Here's how the part is built. I have some questions about the finished solid (model axes, mm). Coordinates: 2 decimals unless noted, no trailing zeros. Order: outer loops, then holes, each group sorted by start corner. A loop starts at its lowest first (then second) coordinate and runs counter-clockwise, first axis right, second up. Notation, with made-up numbers: (17, 9) - (57, 9) arc R18 cw to (57, 27) - close; hole circle Ø1 at (46.25, 73.25). An arc over 180 degrees is marked (long way). Use one line per item in the form item = value. Start each with the question number.
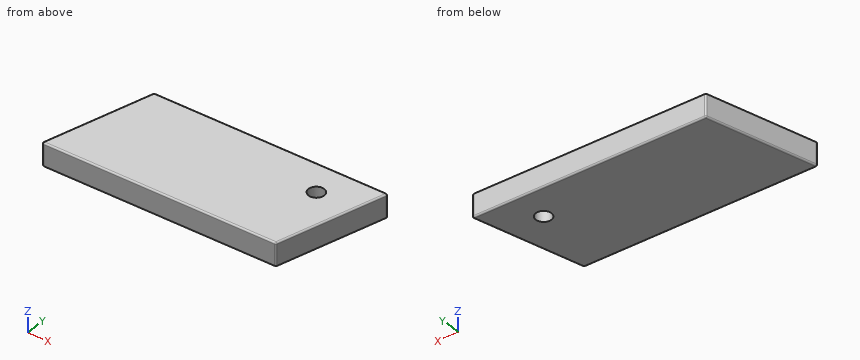
from build123d import *

# Parameters (mm, degrees)
BOSS_EXTRUDE1_DEPTH = 19.05
SKETCH2_R           = 6.35
CUT_EXTRUDE1_DEPTH  = 19.05
FILLET1_R           = 1.27


with BuildPart() as part:
    # Sketch1 → Boss-Extrude1 (new body)
    with BuildSketch(Plane.XY):
        Polygon((0, 0), (23.820683207, 88.9), (214.320683207, 88.9), (190.5, 0), align=None)
    extrude(amount=BOSS_EXTRUDE1_DEPTH)

    # Sketch2 → Cut-Extrude1 (cut)
    with BuildSketch(Plane.XY.offset(19.05)):
        with Locations((176.220683207, 62.083789013)):
            Circle(SKETCH2_R)
    extrude(amount=-CUT_EXTRUDE1_DEPTH, mode=Mode.SUBTRACT)

    # Fillet1
    fillet1_edges = [part.edges().sort_by_distance(p)[0] for p in [
        (119.070683207, 88.9, 19.05),
        (11.910341604, 44.45, 19.05),
        (95.25, 0, 19.05),
        (11.910341604, 44.45, 0),
        (119.070683207, 88.9, 0),
        (202.410341604, 44.45, 0),
        (95.25, 0, 0),
        (0, 0, 9.525),
        (23.820683207, 88.9, 9.525),
        (214.320683207, 88.9, 9.525),
        (190.5, 0, 9.525),
        (202.410341604, 44.45, 19.05),
    ]]
    fillet(fillet1_edges, radius=FILLET1_R)


solid = part.part
1) For pin 1 (1 mm diameter, centred on x = 121.5, y = 37.5, fed in from -Z); pin 2 (8 mm diameter, centred on y = 43, z = 5, fed in from +X); pin 3 (1 mm diameter, centred on y = 23, z = 14, fed in from -X); pin 4 (5 mm diameter, centred on y = 48.5, z = 9, fed in from +X), each with a flat end and sliding along its axis, tell me the tip position at first contact or that it passes through.
2) I need wall thicknesses on probe 1 along X at (y, z) = (58.5, 15); probe 2 along Y at (x, z) = (177, 4); probe 3 along X at (y, z) = (59, 8.25). Which ranges of each line are inside material? Lowest first, please. Write a range as [from, to].
3) Suppose I cut it at B-B, the plane z = 4. List the corners of the cut face in (x, y) for me.
4) Suppose I cut it at A-A, the plane x = 180.5. List the corners of the cut face in (y, z) for me.
From the geometry:
q1.pin_1 = 0
q1.pin_2 = 203.09
q1.pin_3 = 6.03
q1.pin_4 = 204.17
q2.probe_1 = [15.68, 170.98], [181.46, 206.18]
q2.probe_2 = [0, 55.78], [68.39, 88.9]
q2.probe_3 = [15.81, 170.67], [181.77, 206.31]
q3.outline = (0.43, 1.6) arc R1.27 ccw to (1.66, 0) - (189.53, 0) arc R1.27 ccw to (190.75, 0.94) - (213.89, 87.3) arc R1.27 ccw to (212.67, 88.9) - (24.8, 88.9) arc R1.27 ccw to (23.57, 87.96) - close; hole circle Ø12.7 at (176.22, 62.08)
q4.outline = (0, 1.27) arc R1.27 ccw to (1.27, 0) - (57.39, 0) - (57.39, 19.05) - (1.27, 19.05) arc R1.27 ccw to (0, 17.78) - close; (66.78, 0) - (87.63, 0) arc R1.27 ccw to (88.9, 1.27) - (88.9, 17.78) arc R1.27 ccw to (87.63, 19.05) - (66.78, 19.05) - close
